from build123d import *

# Parameters (mm, degrees)
BOSS_EXTRUDE3_DEPTH     = 7
CUT_EXTRUDE1_DEPTH      = 10
SKETCH3_R               = 1.125
CUT_EXTRUDE3_DEPTH      = 1
CUT_EXTRUDE3_DEPTH_BACK = 8
SKETCH4_R               = 1.5
BOSS_EXTRUDE4_DEPTH     = 7
SKETCH5_R               = 1.5
CUT_EXTRUDE4_DEPTH      = 1
CUT_EXTRUDE4_DEPTH_BACK = 8
SKETCH6_R               = 1.125
CUT_EXTRUDE5_DEPTH      = 1
CUT_EXTRUDE5_DEPTH_BACK = 8
CUT_EXTRUDE6_DEPTH      = 1
CUT_EXTRUDE6_DEPTH_BACK = 8


with BuildPart() as part:
    # Sketch1 → Boss-Extrude3 (new body)
    with BuildSketch(Plane(origin=(0, 0, 0), x_dir=(1, 0, 0), z_dir=(0, 1, 0))):
        with BuildLine():
            Line((283.825365173, -12.637997433), (247.825365173, -12.637997433))
            Line((247.825365173, -12.637997433), (247.825365173, -17.637997433))
            ThreePointArc((247.825365173, -17.637997433), (246.360899079, -21.173531339), (242.825365173, -22.637997433))
            Line((242.825365173, -22.637997433), (184.825365173, -22.637997433))
            ThreePointArc((184.825365173, -22.637997433), (181.289831267, -21.173531339), (179.825365173, -17.637997433))
            Line((179.825365173, -17.637997433), (179.825365173, -12.637997433))
            Line((179.825365173, -12.637997433), (143.825365173, -12.637997433))
            ThreePointArc((143.825365173, -12.637997433), (140.289831267, -11.173531339), (138.825365173, -7.637997433))
            Line((138.825365173, -7.637997433), (138.825365173, 20.362002567))
            ThreePointArc((138.825365173, 20.362002567), (140.289831267, 23.897536473), (143.825365173, 25.362002567))
            Line((143.825365173, 25.362002567), (174.825365173, 25.362002567))
            ThreePointArc((174.825365173, 25.362002567), (178.360899079, 26.826468661), (179.825365173, 30.362002567))
            Line((179.825365173, 30.362002567), (179.825365173, 40.362002567))
            ThreePointArc((179.825365173, 40.362002567), (181.289831267, 43.897536473), (184.825365173, 45.362002567))
            Line((184.825365173, 45.362002567), (194.825365173, 45.362002567))
            ThreePointArc((194.825365173, 45.362002567), (198.360899079, 46.826468661), (199.825365173, 50.362002567))
            Line((199.825365173, 50.362002567), (199.825365173, 117.362002567))
            ThreePointArc((199.825365173, 117.362002567), (198.360899079, 120.897536473), (194.825365173, 122.362002567))
            Line((194.825365173, 122.362002567), (184.825365173, 122.362002567))
            ThreePointArc((184.825365173, 122.362002567), (181.289831267, 123.826468661), (179.825365173, 127.362002567))
            Line((179.825365173, 127.362002567), (179.825365173, 132.362002567))
            ThreePointArc((179.825365173, 132.362002567), (181.289831267, 135.897536473), (184.825365173, 137.362002567))
            Line((184.825365173, 137.362002567), (242.825365173, 137.362002567))
            ThreePointArc((242.825365173, 137.362002567), (246.360899079, 135.897536473), (247.825365173, 132.362002567))
            Line((247.825365173, 132.362002567), (247.825365173, 127.362002567))
            ThreePointArc((247.825365173, 127.362002567), (246.360899079, 123.826468661), (242.825365173, 122.362002567))
            Line((242.825365173, 122.362002567), (232.825365173, 122.362002567))
            ThreePointArc((232.825365173, 122.362002567), (229.289831267, 120.897536473), (227.825365173, 117.362002567))
            Line((227.825365173, 117.362002567), (227.825365173, 50.362002567))
            ThreePointArc((227.825365173, 50.362002567), (229.289831267, 46.826468661), (232.825365173, 45.362002567))
            Line((232.825365173, 45.362002567), (242.825365173, 45.362002567))
            ThreePointArc((242.825365173, 45.362002567), (246.360899079, 43.897536473), (247.825365173, 40.362002567))
            Line((247.825365173, 40.362002567), (247.825365173, 30.362002567))
            ThreePointArc((247.825365173, 30.362002567), (249.289831267, 26.826468661), (252.825365173, 25.362002567))
            Line((252.825365173, 25.362002567), (283.825365173, 25.362002567))
            ThreePointArc((283.825365173, 25.362002567), (287.360899079, 23.897536473), (288.825365173, 20.362002567))
            Line((288.825365173, 20.362002567), (288.825365173, -7.637997433))
            ThreePointArc((288.825365173, -7.637997433), (287.360899079, -11.173531339), (283.825365173, -12.637997433))
        make_face()
    extrude(amount=BOSS_EXTRUDE3_DEPTH)

    # Sketch2 → Cut-Extrude1 (cut)
    with BuildSketch(Plane(origin=(0, 7, 0), x_dir=(1, 0, 0), z_dir=(0, 1, 0))):
        with BuildLine():
            Line((179.825365173, -12.637997433), (247.825365173, -12.637997433))
            Line((247.825365173, -12.637997433), (247.825365173, -17.637997433))
            ThreePointArc((247.825365173, -17.637997433), (246.360899079, -21.173531339), (242.825365173, -22.637997433))
            Line((242.825365173, -22.637997433), (184.825365173, -22.637997433))
            ThreePointArc((184.825365173, -22.637997433), (181.289831267, -21.173531339), (179.825365173, -17.637997433))
            Line((179.825365173, -17.637997433), (179.825365173, -12.637997433))
        make_face()
    extrude(amount=-CUT_EXTRUDE1_DEPTH, mode=Mode.SUBTRACT)

    # Sketch3 → Cut-Extrude3 (cut, two sides)
    with BuildSketch(Plane(origin=(0, 7, 0), x_dir=(1, 0, 0), z_dir=(0, 1, 0))) as cut_extrude3_sk:
        with Locations((143.075365173, 15.362002567)):
            Circle(SKETCH3_R)
        with Locations((143.075365173, -2.637997433)):
            Circle(SKETCH3_R)
        with Locations((284.575365173, -2.637997433)):
            Circle(SKETCH3_R)
        with Locations((284.575365173, 15.362002567)):
            Circle(SKETCH3_R)
        with BuildLine():
            Line((236.729776069, 25.219549299), (236.729776069, 4.789235296))
            ThreePointArc((236.729776069, 4.789235296), (233.800843881, -2.281832516), (226.729776069, -5.210764704))
            Line((226.729776069, -5.210764704), (200.920954278, -5.210764704))
            ThreePointArc((200.920954278, -5.210764704), (193.849886466, -2.281832516), (190.920954278, 4.789235296))
            Line((190.920954278, 4.789235296), (190.920954278, 25.219549299))
            ThreePointArc((190.920954278, 25.219549299), (193.849886466, 32.290617111), (200.920954278, 35.219549299))
            Line((200.920954278, 35.219549299), (226.729776069, 35.219549299))
            ThreePointArc((226.729776069, 35.219549299), (233.800843881, 32.290617111), (236.729776069, 25.219549299))
        make_face()
    extrude(amount=CUT_EXTRUDE3_DEPTH, mode=Mode.SUBTRACT)
    extrude(cut_extrude3_sk.sketch, amount=-CUT_EXTRUDE3_DEPTH_BACK, mode=Mode.SUBTRACT)

    # Sketch4 → Boss-Extrude4 (add)
    with BuildSketch(Plane(origin=(0, 7, 0), x_dir=(1, 0, 0), z_dir=(0, 1, 0))):
        with BuildLine():
            Line((233.679703761, 121.865339942), (243.89819588, 121.865339942))
            Line((243.89819588, 121.865339942), (253.825365173, 128.052186148))
            Line((253.825365173, 128.052186148), (253.825365173, 137.362002567))
            Line((253.825365173, 137.362002567), (173.825365173, 137.362002567))
            Line((173.825365173, 137.362002567), (173.825365173, 128.052186148))
            Line((173.825365173, 128.052186148), (183.752534467, 121.865339942))
            Line((183.752534467, 121.865339942), (193.971026586, 121.865339942))
            ThreePointArc((193.971026586, 121.865339942), (198.282425053, 116.602256541), (199.825365173, 109.975980106))
            Line((199.825365173, 109.975980106), (199.825365173, 83.862002567))
            Line((199.825365173, 83.862002567), (227.825365173, 83.862002567))
            Line((227.825365173, 83.862002567), (227.825365173, 109.975980106))
            ThreePointArc((227.825365173, 109.975980106), (229.368305294, 116.602256541), (233.679703761, 121.865339942))
        make_face()
        with Locations((183.89819588, 129.862002567)):
            Circle(SKETCH4_R, mode=Mode.SUBTRACT)
        with Locations((243.89819588, 129.862002567)):
            Circle(SKETCH4_R, mode=Mode.SUBTRACT)
    extrude(amount=-BOSS_EXTRUDE4_DEPTH)

    # Sketch5 → Cut-Extrude4 (cut, two sides)
    with BuildSketch(Plane(origin=(0, 7, 0), x_dir=(1, 0, 0), z_dir=(0, 1, 0))) as cut_extrude4_sk:
        with Locations((183.825365173, 130.832171384)):
            Circle(SKETCH5_R)
        with Locations((243.825365173, 130.832171384)):
            Circle(SKETCH5_R)
        with Locations((242.825365173, 40.362002567)):
            Circle(SKETCH5_R)
        with Locations((184.825365173, 40.362002567)):
            Circle(SKETCH5_R)
        with Locations((184.825365173, -5.210764704)):
            Circle(SKETCH5_R)
        with Locations((242.825365173, -5.210764704)):
            Circle(SKETCH5_R)
    extrude(amount=CUT_EXTRUDE4_DEPTH, mode=Mode.SUBTRACT)
    extrude(cut_extrude4_sk.sketch, amount=-CUT_EXTRUDE4_DEPTH_BACK, mode=Mode.SUBTRACT)

    # Sketch6 → Cut-Extrude5 (cut, two sides)
    with BuildSketch(Plane(origin=(0, 7, 0), x_dir=(1, 0, 0), z_dir=(0, 1, 0))) as cut_extrude5_sk:
        with Locations((284.575365173, 15.362002567)):
            Circle(SKETCH6_R)
        with Locations((213.825365173, 96.329183022)):
            Circle(SKETCH6_R)
        with Locations((213.825365173, 114.177699089)):
            Circle(SKETCH6_R)
    extrude(amount=CUT_EXTRUDE5_DEPTH, mode=Mode.SUBTRACT)
    extrude(cut_extrude5_sk.sketch, amount=-CUT_EXTRUDE5_DEPTH_BACK, mode=Mode.SUBTRACT)

    # Sketch7 → Cut-Extrude6 (cut, two sides)
    with BuildSketch(Plane(origin=(0, 7, 0), x_dir=(1, 0, 0), z_dir=(0, 1, 0))) as cut_extrude6_sk:
        with BuildLine():
            Line((193.971026586, 134.106855399), (233.679703761, 134.106855399))
            ThreePointArc((233.679703761, 134.106855399), (238.2529795, 129.533579659), (233.679703761, 124.96030392))
            Line((233.679703761, 124.96030392), (193.971026586, 124.96030392))
            ThreePointArc((193.971026586, 124.96030392), (189.397750847, 129.533579659), (193.971026586, 134.106855399))
        make_face()
    extrude(amount=CUT_EXTRUDE6_DEPTH, mode=Mode.SUBTRACT)
    extrude(cut_extrude6_sk.sketch, amount=-CUT_EXTRUDE6_DEPTH_BACK, mode=Mode.SUBTRACT)


solid = part.part
Read the model definition and answer for the solid it produces. Units are mm, in the model's axes. A direction names the side the tool comes from. Coordinates: 2 decimals unless noted, no trailing zeros. Loops run counter-clockwise (first coordinate to the right, second up) from the corner with the lowest first, then second, coordinate; pieces in that order, holes last. Notation, with made-up numbers: (-16, -3) -> (19, -3) arc R20 cw to (19, 25) -> close; hole circle Ø1 at (86, -21.5). An arc over 180 degrees is marked (long way). Write item = value, one per line. Start each with the question number.
1) The mould has two halves that part along X. Classify faces 1 (the face through (229.251, 3.451, -46.866)), 2 (the face through (238.25, 3.55, -129.63)), 3 (the face through (138.825, 3, -6)): pulls with the +X half, pulls with the -X half, needs draft (parallel to the pull), parting line crosses it, or undercut.
2) The part is cut by section C-C, the plane x = 165. Determine the outline of the cut face in (y, z), plus the area to 3 significant figures.
3) The part is cut by section A-A, the plane z = -7.5. Determine the outline of the cut face in (x, y), plus the area to 3 significant figures.
4) The part is cut by section D-D, the plane z = -74. Determine the outline of the cut face in (x, y), plus the area to 3 significant figures.
5) The part is cut by section B-B, the plane x = 210.5. Determine the outline of the cut face in (y, z), plus the area to 3 significant figures.
6) Given P1, Ø2, axis at y = 4.5, z = -35.5, coming from the +X side; P2, Ø1, axis at x = 257, y = 3.5, coming from the -Z side; P3, Ø2, axis at y = 2.5, z = -54.5, coming from the +X side, each flat-ended and moving along its own axis, determine where each tip first touches the part or whether it passes through.
7) Find the intervals of material crossed by L1, parallel to Z at x = 202.5, y = 4.5; L2, parallel to X at y = 0.5, z = -17; L3, parallel to X at y = 5, z = -39, in increasing order. Write a range as from..to.
8) For faces 4 (the face through (173.825, 4, -133)), 5 (the face through (189.4, 3.5, -129.4)), 6 (the face through (248.792, 3.549, -124.915)), determine the directions among +Z, -Z, +X, -X, +Y, -Y from which every point of the face is accessible in a straight line to the end or side of a thin tool.
Result:
q1.face_1 = pulls with the +X half
q1.face_2 = undercut
q1.face_3 = pulls with the -X half
q2.outline = (0, -25.36) -> (7, -25.36) -> (7, 12.64) -> (0, 12.64) -> close
q2.area = 266 mm²
q3.outline = (138.83, 0) -> (190.92, 0) -> (190.92, 7) -> (138.83, 7) -> close; (236.73, 0) -> (288.83, 0) -> (288.83, 7) -> (236.73, 7) -> close
q3.area = 729 mm²
q4.outline = (199.83, 0) -> (227.83, 0) -> (227.83, 7) -> (199.83, 7) -> close
q4.area = 196 mm²
q5.outline = (0, -137.36) -> (7, -137.36) -> (7, -134.11) -> (0, -134.11) -> close; (0, -124.96) -> (7, -124.96) -> (7, -35.22) -> (0, -35.22) -> close; (0, 5.21) -> (7, 5.21) -> (7, 12.64) -> (0, 12.64) -> close
q5.area = 703 mm²
q6.P1 = 247.83
q6.P2 = -25.36
q6.P3 = 227.83
q7.L1 = -137.36..-134.11, -124.96..-35.22, 5.21..12.64
q7.L2 = 138.83..190.92, 236.73..288.83
q7.L3 = 179.83..184.2, 185.45..242.2, 243.45..247.83
q8.face_4 = -Z, -X, +Y, -Y
q8.face_5 = +Y, -Y
q8.face_6 = +X, +Y, -Y
